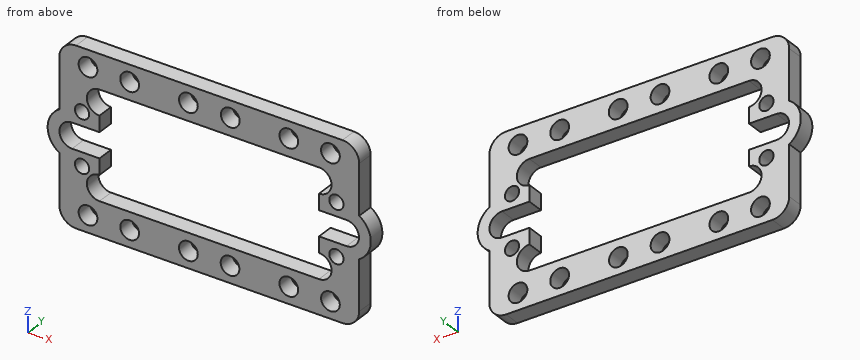
```python
from build123d import *

# Parameters (mm, degrees)
MASS_DEPTH               = 3.175
SKETCH2_W                = 41.656
SKETCH2_H                = 4.7625
SERVO_HOLE_DEPTH         = 4.175
F_6_32_SERVO_MOUNT_D     = 2.7051
F_6_32_SERVO_MOUNT_DEPTH = 152.4
F_6_32_SERVO_MOUNT_TIP   = 0.81269403
CORNERS_R                = 3.175
SKETCH5_R                = 1.778
MOUNTING_HOLES_DEPTH     = 4.175


with BuildPart() as part:
    # Sketch1 → Mass (new body)
    with BuildSketch(Plane(origin=(0, 0, 0), x_dir=(1, 0, 0), z_dir=(0, 1, 0))):
        with BuildLine():
            Line((-28.448, 16.637), (28.448, 16.637))
            Line((28.448, 16.637), (28.448, 3.943058564))
            ThreePointArc((28.448, 3.943058564), (30.6578, 0), (28.448, -3.943058564))
            Line((28.448, -3.943058564), (28.448, -16.637))
            Line((28.448, -16.637), (-28.448, -16.637))
            Line((-28.448, -16.637), (-28.448, -3.943058564))
            ThreePointArc((-28.448, -3.943058564), (-30.6578, 0), (-28.448, 3.943058564))
            Line((-28.448, 3.943058564), (-28.448, 16.637))
        make_face()
    extrude(amount=MASS_DEPTH)

    # Sketch2 → Servo Hole (cut, through all)
    with BuildSketch(Plane(origin=(0, 3.175, 0), x_dir=(1, 0, 0), z_dir=(0, 1, 0))):
        with BuildLine():
            ThreePointArc((-20.828, -5.3975), (-23.20925, -7.77875), (-20.828, -10.16))
            Line((-20.828, -10.16), (20.828, -10.16))
            ThreePointArc((20.828, -10.16), (23.20925, -7.77875), (20.828, -5.3975))
            Line((20.828, -5.3975), (20.828, -2.38125))
            Line((20.828, -2.38125), (-20.828, -2.38125))
            Line((-20.828, -2.38125), (-20.828, -5.3975))
        make_face()
        Rectangle(SKETCH2_W, SKETCH2_H)
        with BuildLine():
            Line((-20.828, 5.3975), (-20.828, 2.38125))
            Line((-20.828, 2.38125), (20.828, 2.38125))
            Line((20.828, 2.38125), (20.828, 5.3975))
            ThreePointArc((20.828, 5.3975), (23.20925, 7.77875), (20.828, 10.16))
            Line((20.828, 10.16), (-20.828, 10.16))
            ThreePointArc((-20.828, 10.16), (-23.20925, 7.77875), (-20.828, 5.3975))
        make_face()
        with BuildLine():
            Line((20.828, 2.38125), (20.828, -2.38125))
            Line((20.828, -2.38125), (26.035, -2.38125))
            ThreePointArc((26.035, -2.38125), (28.41625, 0), (26.035, 2.38125))
            Line((26.035, 2.38125), (20.828, 2.38125))
        make_face()
        with BuildLine():
            Line((-26.035, -2.38125), (-20.828, -2.38125))
            Line((-20.828, -2.38125), (-20.828, 2.38125))
            Line((-20.828, 2.38125), (-26.035, 2.38125))
            ThreePointArc((-26.035, 2.38125), (-28.41625, 0), (-26.035, -2.38125))
        make_face()
    extrude(amount=-SERVO_HOLE_DEPTH, mode=Mode.SUBTRACT)

    # #6-32 Servo Mount
    with Locations(Plane(origin=(0, 3.175, 0), x_dir=(1, 0, 0), z_dir=(0, 1, 0))):
        with Locations((24.13, 4.953), (24.13, -4.953), (-24.13, -4.953), (-24.13, 4.953)):
            Hole(F_6_32_SERVO_MOUNT_D / 2, depth=F_6_32_SERVO_MOUNT_DEPTH)
            with Locations((0, 0, -(F_6_32_SERVO_MOUNT_DEPTH + F_6_32_SERVO_MOUNT_TIP / 2))):  # 118° drill point
                Cone(0, F_6_32_SERVO_MOUNT_D / 2, F_6_32_SERVO_MOUNT_TIP, mode=Mode.SUBTRACT)

    # Corners
    corners_edges = [part.edges().sort_by_distance(p)[0] for p in [
        (-28.448, 1.5875, -16.637),
        (28.448, 1.5875, -16.637),
        (28.448, 1.5875, 16.637),
        (-28.448, 1.5875, 16.637),
    ]]
    fillet(corners_edges, radius=CORNERS_R)

    # Sketch5 → Mounting Holes (cut, through all)
    with BuildSketch(Plane(origin=(0, 3.175, 0), x_dir=(1, 0, 0), z_dir=(0, 1, 0))):
        with Locations((-22.9997, 13.4747)):
            Circle(SKETCH5_R)
        with Locations((22.9997, 13.4747)):
            Circle(SKETCH5_R)
        with Locations((22.9997, -13.4747)):
            Circle(SKETCH5_R)
        with Locations((-22.9997, -13.4747)):
            Circle(SKETCH5_R)
        with Locations((-15.1003, 13.4747)):
            Circle(SKETCH5_R)
        with Locations((-3.9497, 13.4747)):
            Circle(SKETCH5_R)
        with Locations((3.9497, 13.4747)):
            Circle(SKETCH5_R)
        with Locations((15.1003, 13.4747)):
            Circle(SKETCH5_R)
        with Locations((15.1003, -13.4747)):
            Circle(SKETCH5_R)
        with Locations((4.0005, -13.4747)):
            Circle(SKETCH5_R)
        with Locations((-3.9497, -13.4747)):
            Circle(SKETCH5_R)
        with Locations((-15.1003, -13.4747)):
            Circle(SKETCH5_R)
    extrude(amount=-MOUNTING_HOLES_DEPTH, mode=Mode.SUBTRACT)


solid = part.part
```
Design review of the part built by this model. Coordinates are the model's own, in mm. Round coordinates to 2 decimals unless told otherwise and drop trailing zeros. Write each loop counter-clockwise with the first axis right and the second up, starting at its lowest first coordinate (ties: lowest second). Pieces come first, ordered by that corner, then holes.
Item 1: We need section B-B on x = -8.5. Write out the cut boundary in (y, z) (3 decimals), and give its area (3 significant figures).
Item 2: Clearance check with flat-ended pins moving along their axes: pin 1 Ø1 at (x, z) = (-1.5, 9.5) entering from +Y; pin 2 Ø1.6 at (y, z) = (1.5, 9.5) entering from +X; pin 3 Ø1 at (y, z) = (1.5, -11) entering from -X. State where each tip first meets the part, or that it passes through.
Item 3: We need section A-A on z = 0. Write out the cut boundary in (x, y) (3 decimals).
Item 4: For probe 1 along Z at (x, y) = (-15, 2.5); probe 2 along Z at (x, y) = (18.5, 2.25); probe 3 along X at (y, z) = (2.05, -8), list the stretches that pass through material, from the lowest coordinate up.
Item 5: We need section D-D on y = 1.3. State how many separate pieces and enclosed holes the cut face has, and give its area (3 significant figures).
Item 6: We need section C-C on x = -24.13. Write out the cut boundary in (y, z) (3 decimals).
Returned:
1. outline: (0, -16.637) - (3.175, -16.637) - (3.175, -10.16) - (0, -10.16) - close; (0, 10.16) - (3.175, 10.16) - (3.175, 16.637) - (0, 16.637) - close
1. area: 41.1 mm2
2. pin 1: passes through
2. pin 2: stops at x = 28.45
2. pin 3: stops at x = -28.45
3. outline: (-30.658, 0) - (-28.416, 0) - (-28.416, 3.175) - (-30.658, 3.175) - close; (28.416, 0) - (30.658, 0) - (30.658, 3.175) - (28.416, 3.175) - close
4. probe 1: z = -16.64 to -15.25, -11.7 to -10.16, 10.16 to 11.7, 15.25 to 16.64
4. probe 2: z = -16.64 to -10.16, 10.16 to 16.64
4. probe 3: x = -28.45 to -23.2, 23.2 to 28.45
5. separate pieces: 1
5. enclosed holes: 17
5. area: 817 mm2
6. outline: (0, -16.637) - (3.175, -16.637) - (3.175, -14.847) - (0, -14.847) - close; (0, -12.102) - (3.175, -12.102) - (3.175, -6.306) - (0, -6.306) - close; (0, -3.6) - (3.175, -3.6) - (3.175, -2.381) - (0, -2.381) - close; (0, 2.381) - (3.175, 2.381) - (3.175, 3.6) - (0, 3.6) - close; (0, 6.306) - (3.175, 6.306) - (3.175, 12.102) - (0, 12.102) - close; (0, 14.847) - (3.175, 14.847) - (3.175, 16.637) - (0, 16.637) - close
